```python
from build123d import *

# Parameters (mm, degrees)
CASEENVELOPE_W                       = 92
CASEENVELOPE_H                       = 63
BOTTOM_ENVELOPE_DEPTH                = 8
OUTSIDE_R3_R                         = 3
SHELL_1_T                            = -2
SIDEPORT_CLEARANCE_1_START           = 6.45
SIDEPORT_PROFILE_1_W                 = 10.1
SIDEPORT_PROFILE_1_H                 = 13
SIDEPORT_CLEARANCE_1_DEPTH           = 4.5
SIDEPORT_CLEARANCE_2_START           = 6.45
SIDEPORT_PROFILE_2_W                 = 7.7
SIDEPORT_PROFILE_2_H                 = 13
SIDEPORT_CLEARANCE_2_DEPTH           = 4.7
SIDEPORT_CLEARANCE_3_START           = 6.45
SIDEPORT_PROFILE_3_W                 = 7.7
SIDEPORT_PROFILE_3_H                 = 13
SIDEPORT_CLEARANCE_3_DEPTH           = 4.7
ENDPORT_CLEARANCE_1_START            = 6.45
ENDPORT_PROFILE_1_W                  = 11
ENDPORT_PROFILE_1_H                  = 17.3
ENDPORT_CLEARANCE_1_DEPTH            = 14.6
ENDPORT_CLEARANCE_2_START            = 6.45
ENDPORT_PROFILE_2_W                  = 11
ENDPORT_PROFILE_2_H                  = 14.7
ENDPORT_CLEARANCE_2_DEPTH            = 16.3
ENDPORT_CLEARANCE_3_START            = 6.45
ENDPORT_PROFILE_3_W                  = 11
ENDPORT_PROFILE_3_H                  = 14.7
ENDPORT_CLEARANCE_3_DEPTH            = 16.3
FOUR_M2P5_STANDOFFS_2P05_PILOT_START = 2
STANDOFF_RINGS_R                     = 2.75
STANDOFF_RINGS_R_2                   = 1.025
FOUR_M2P5_STANDOFFS_2P05_PILOT_DEPTH = 3.5


with BuildPart() as part:
    # CaseEnvelope → Bottom_Envelope (new body)
    with BuildSketch(Plane.XY):
        Rectangle(CASEENVELOPE_W, CASEENVELOPE_H)
    extrude(amount=BOTTOM_ENVELOPE_DEPTH)

    # Outside_R3
    outside_r3_edges = [part.edges().sort_by_distance(p)[0] for p in [
        (46, -31.5, 4),
        (-46, -31.5, 4),
        (-46, 31.5, 4),
        (46, 31.5, 4),
    ]]
    fillet(outside_r3_edges, radius=OUTSIDE_R3_R)

    # 抽壳1
    shell_1_openings = [part.faces().sort_by_distance(p)[0] for p in [
        (0, 0, 8),
    ]]
    offset(amount=SHELL_1_T, openings=shell_1_openings, kind=Kind.INTERSECTION)

    # SidePort_Profile_1 → SidePort_Clearance_1 (cut)
    with BuildSketch(Plane.XY.offset(SIDEPORT_CLEARANCE_1_START)):
        with Locations((-31.3, -33.5)):
            Rectangle(SIDEPORT_PROFILE_1_W, SIDEPORT_PROFILE_1_H)
    extrude(amount=SIDEPORT_CLEARANCE_1_DEPTH, mode=Mode.SUBTRACT)

    # SidePort_Profile_2 → SidePort_Clearance_2 (cut)
    with BuildSketch(Plane.XY.offset(SIDEPORT_CLEARANCE_2_START)):
        with Locations((-16.7, -33.5)):
            Rectangle(SIDEPORT_PROFILE_2_W, SIDEPORT_PROFILE_2_H)
    extrude(amount=SIDEPORT_CLEARANCE_2_DEPTH, mode=Mode.SUBTRACT)

    # SidePort_Profile_3 → SidePort_Clearance_3 (cut)
    with BuildSketch(Plane.XY.offset(SIDEPORT_CLEARANCE_3_START)):
        with Locations((-3.3, -33.5)):
            Rectangle(SIDEPORT_PROFILE_3_W, SIDEPORT_PROFILE_3_H)
    extrude(amount=SIDEPORT_CLEARANCE_3_DEPTH, mode=Mode.SUBTRACT)

    # EndPort_Profile_1 → EndPort_Clearance_1 (cut)
    with BuildSketch(Plane.XY.offset(ENDPORT_CLEARANCE_1_START)):
        with Locations((47.5, -17.8)):
            Rectangle(ENDPORT_PROFILE_1_W, ENDPORT_PROFILE_1_H)
    extrude(amount=ENDPORT_CLEARANCE_1_DEPTH, mode=Mode.SUBTRACT)

    # EndPort_Profile_2 → EndPort_Clearance_2 (cut)
    with BuildSketch(Plane.XY.offset(ENDPORT_CLEARANCE_2_START)):
        with Locations((47.5, 1.1)):
            Rectangle(ENDPORT_PROFILE_2_W, ENDPORT_PROFILE_2_H)
    extrude(amount=ENDPORT_CLEARANCE_2_DEPTH, mode=Mode.SUBTRACT)

    # EndPort_Profile_3 → EndPort_Clearance_3 (cut)
    with BuildSketch(Plane.XY.offset(ENDPORT_CLEARANCE_3_START)):
        with Locations((47.5, 19)):
            Rectangle(ENDPORT_PROFILE_3_W, ENDPORT_PROFILE_3_H)
    extrude(amount=ENDPORT_CLEARANCE_3_DEPTH, mode=Mode.SUBTRACT)

    # Standoff_Rings → Four_M2p5_Standoffs_2p05_Pilot (add)
    # profile 1 of 4: a face of its own
    with BuildSketch(Plane.XY.offset(FOUR_M2P5_STANDOFFS_2P05_PILOT_START)):
        with Locations(Location((-39, -24.5, 0), (0, 0, 180))):
            Circle(STANDOFF_RINGS_R)
        with Locations((-39, -24.5)):
            Circle(STANDOFF_RINGS_R_2, mode=Mode.SUBTRACT)
    # profile 2 of 4: a face of its own
    with BuildSketch(Plane.XY.offset(FOUR_M2P5_STANDOFFS_2P05_PILOT_START)):
        with Locations(Location((-39, 24.5, 0), (0, 0, 180))):
            Circle(STANDOFF_RINGS_R)
        with Locations((-39, 24.5)):
            Circle(STANDOFF_RINGS_R_2, mode=Mode.SUBTRACT)
    # profile 3 of 4: a face of its own
    with BuildSketch(Plane.XY.offset(FOUR_M2P5_STANDOFFS_2P05_PILOT_START)):
        with Locations(Location((19, -24.5, 0), (0, 0, 180))):
            Circle(STANDOFF_RINGS_R)
        with Locations((19, -24.5)):
            Circle(STANDOFF_RINGS_R_2, mode=Mode.SUBTRACT)
    # profile 4 of 4: a face of its own
    with BuildSketch(Plane.XY.offset(FOUR_M2P5_STANDOFFS_2P05_PILOT_START)):
        with Locations(Location((19, 24.5, 0), (0, 0, 180))):
            Circle(STANDOFF_RINGS_R)
        with Locations((19, 24.5)):
            Circle(STANDOFF_RINGS_R_2, mode=Mode.SUBTRACT)
    extrude(amount=FOUR_M2P5_STANDOFFS_2P05_PILOT_DEPTH)


solid = part.part
```
Verification items for the finished model (mm, model axes). A direction names the side the tool comes from. Coordinates: 2 decimals unless noted, no trailing zeros. Order: outer loops, then holes, each group sorted by start corner. A loop starts at its lowest first (then second) coordinate and runs counter-clockwise, first axis right, second up. Notation, with made-up numbers: (87, 86.5) - (128, 86.5) arc R32 cw to (128, 121.5) - close; hole circle Ø2 at (31, -17). An arc over 180 degrees is marked (long way). Return JSON: item names as keys, results as strings.
(1) Mould release check, pull along Y, two halves, no side actions. Record for faces 1 (the flat face through (45, 10, 8)), 2 (the cylindrical face through (-45.14, -30.6, 4.06)), 3 (the flat face through (45, -18, 6.45)): pulls with the +Y half, pulls with the -Y half, needs draft (parallel to the pull), parting line crosses it, or undercut.
Filled sheet:
{"face 1": "needs draft", "face 2": "pulls with the -Y half", "face 3": "undercut"}
(2) Section check C-C, the plane y = 24.5. Record the cut outline in (x, z) (3 decimals), and give its area (3 significant figures).
Filled sheet:
{"outline": "(-46, 0) - (46, 0) - (46, 6.45) - (44, 6.45) - (44, 2) - (21.75, 2) - (21.75, 5.5) - (20.025, 5.5) - (20.025, 2) - (17.975, 2) - (17.975, 5.5) - (16.25, 5.5) - (16.25, 2) - (-36.25, 2) - (-36.25, 5.5) - (-37.975, 5.5) - (-37.975, 2) - (-40.025, 2) - (-40.025, 5.5) - (-41.75, 5.5) - (-41.75, 2) - (-44, 2) - (-44, 8) - (-46, 8) - close", "area": "229 mm^2"}
(3) Thickness scan on line 1 along Y through (x, z) = (-39, 4.05) (3 decimals); line 2 along Y through (x, z) = (-16.5, 5.75); line 3 along X through (y, z) = (7.5, 5). Record the ranges inside material, lowest first.
Filled sheet:
{"line 1": "y = -31.5 to -29.5, -27.25 to -25.525, -23.475 to -21.75, 21.75 to 23.475, 25.525 to 27.25, 29.5 to 31.5", "line 2": "y = -31.5 to -29.5, 29.5 to 31.5", "line 3": "x = -46 to -44, 44 to 46"}
(4) Go/stop test with flat-tipped pins: pin 1 (0.5 mm diameter, centred on y = -30, z = 7.5, fed in from -X); pin 2 (1.7 mm diameter, centred on y = -30.5, z = 7, fed in from +X); pin 3 (4.5 mm diameter, centred on x = -38.5, y = -25.5, fed in from +Z). Record where each tip stops, or that it passes through.
Filled sheet:
{"pin 1": "stops at x = -45.73", "pin 2": "stops at x = 45.77", "pin 3": "stops at z = 5.5"}
(5) Section check A-A, the plane y = -13. Record the cut outline in (x, z).
Filled sheet:
{"outline": "(-46, 0) - (46, 0) - (46, 6.45) - (44, 6.45) - (44, 2) - (-44, 2) - (-44, 8) - (-46, 8) - close"}
(6) Section check D-D, the plane x = -39. Record the cut outline in (y, z) (3 decimals).
Filled sheet:
{"outline": "(-31.5, 0) - (31.5, 0) - (31.5, 8) - (29.5, 8) - (29.5, 2) - (27.25, 2) - (27.25, 5.5) - (25.525, 5.5) - (25.525, 2) - (23.475, 2) - (23.475, 5.5) - (21.75, 5.5) - (21.75, 2) - (-21.75, 2) - (-21.75, 5.5) - (-23.475, 5.5) - (-23.475, 2) - (-25.525, 2) - (-25.525, 5.5) - (-27.25, 5.5) - (-27.25, 2) - (-29.5, 2) - (-29.5, 8) - (-31.5, 8) - close"}
(7) Access from +Z, -Z, +X, -X, +Y, -Y to the whole of each face (thin tool, end or side, straight path). Record for faces 4 (the flat face through (19, 26, 5.5)), 5 (the cylindrical face through (-45.14, 30.6, 4.06)).
Filled sheet:
{"face 4": "+Z", "face 5": "+Z, -Z, -X, +Y"}
(8) Section check B-B, the plane x = -29. Record the cut outline in (y, z), and give its area (3 significant figures).
Filled sheet:
{"outline": "(-31.5, 0) - (31.5, 0) - (31.5, 8) - (29.5, 8) - (29.5, 2) - (-29.5, 2) - (-29.5, 6.45) - (-31.5, 6.45) - close", "area": "147 mm^2"}
